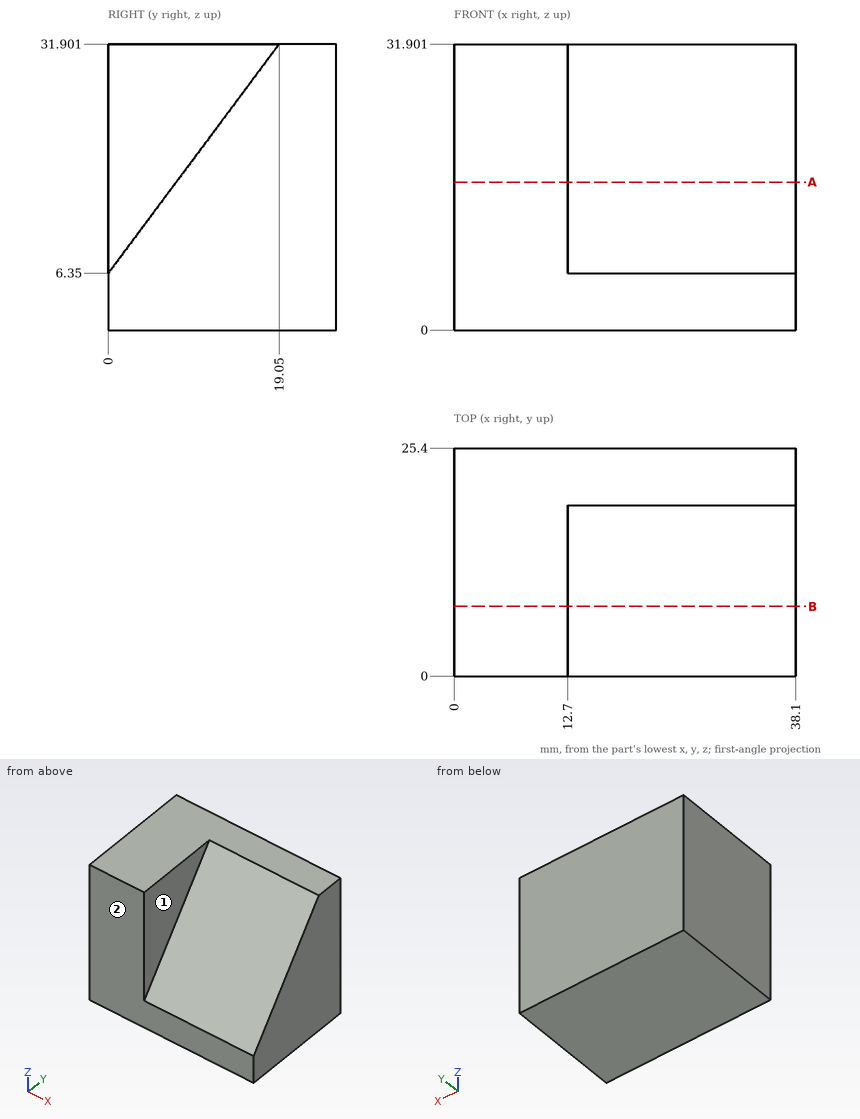
The figure shows three views and two pictorial views of one solid part (mm, origin at its lowest corner). Answer the questions. A direction names the side the tool comes from. Round coordinates to 2 decimals unless told otherwise and drop trailing zeros. Order: outer loops, then holes, each group sorted by start corner. A loop starts at its lowest first (then second) coordinate and runs counter-clockwise, first axis right, second up. Notation, with made-up numbers: M 86.5,58 L 118.5,58 A26 cw 118.5,90 Z; hole C 51,-29 d8. An arc over 180 degrees is marked long. Put each result on its own line as item: value. Start each with the question number.
Q1. Section A-A, the plane z = 16.5 is taken. Write down the section's boundary in (x, y).
Q2. Section B-B, the plane y = 7.75 is taken. Write down the section's boundary in (x, z) (1 decimal).
Q3. Flat-ended cylindrical pins translate along their axes: pin 1 (10 mm diameter, centred on x = 27, y = 9, fed in from +Z); pin 2 (3 mm diameter, centred on y = 11, z = 28, fed in from +X); pin 3 (3 mm diameter, centred on x = 17, z = 9.5, fed in from -Y); pin 4 (5 mm diameter, centred on x = 6.5, y = 11.5, fed in from -Z). Find the tip coordinate at first contact, or state that the pin passes through.
Q4. A tool of negligible diameter and unlimited length cuts with its end or side. For the marked faces 1 and 2, from which of +Z, -Z, +X, -X, +Y, -Y can it reach the whole face along a straight path? Write none if from no direction.
Q5. Straight lines are drawn through the part: L1, parallel to X at y = 4.5, z = 15.5; L2, parallel to Y at x = 17.5, z = 17.5; L3, parallel to Z at x = 31, y = 8.5. For each, find the intervals that lie inside material, in ascending order. Write a range as [from, to].
Findings below:
1. outline: M 0,0 L 12.7,0 L 12.7,7.57 L 38.1,7.57 L 38.1,25.4 L 0,25.4 Z
2. outline: M 0,0 L 38.1,0 L 38.1,16.7 L 12.7,16.7 L 12.7,31.9 L 0,31.9 Z
3. pin 1: stops at z = 25.13
3. pin 2: stops at x = 12.7
3. pin 3: stops at y = 1.23
3. pin 4: stops at z = 0
4. face 1: +Z, +X, -Y
4. face 2: +Z, -Z, +X, -X, -Y
5. L1: x = [0, 12.7]
5. L2: y = [8.31, 25.4]
5. L3: z = [0, 17.75]
